```python
from build123d import *

# Parameters (mm, degrees)
SKETCH1_R           = 0.627
BOSS_EXTRUDE1_DEPTH = 0.762
FILLET1_R           = 2.54
FILLET2_RADIUS      = 0.5039995
FILLET2_LENGTH      = 0.762


with BuildPart() as part:
    # Sketch1 → Boss-Extrude1 (new body)
    with BuildSketch(Plane.XY):
        with BuildLine():
            Line((-0.508, -9.511443686), (-0.508, -17.4625))
            Line((-0.508, -17.4625), (0.499999, -17.4625))
            Line((0.499999, -17.4625), (0.499999, -9.51186764))
            ThreePointArc((0.499999, -9.51186764), (0.004006112, 9.524999158), (-0.508, -9.511443686))
        make_face()
        Circle(SKETCH1_R, mode=Mode.SUBTRACT)
    extrude(amount=BOSS_EXTRUDE1_DEPTH)

    # Fillet1
    fillet1_edges = [part.edges().sort_by_distance(p)[0] for p in [
        (0.499999, -9.51186764, 0.381),
        (-0.508, -9.511443686, 0.381),
    ]]
    fillet(fillet1_edges, radius=FILLET1_R)

    # Fillet2: full round fillet: the end face becomes a half cylinder, R = half its width
    fillet2_face = Plane((-0.0040005, -17.4625, 0.381), x_dir=(0, 0, 1), z_dir=(0, -1, 0))  # on the end face: x along it, z out of the body
    fillet2_slab = fillet2_face.offset(-FILLET2_RADIUS / 2) * Box(FILLET2_LENGTH, 2 * FILLET2_RADIUS, FILLET2_RADIUS, mode=Mode.PRIVATE)  # the body's end, R deep
    fillet2_round = Plane((-0.0040005, -16.9585005, 0.381), x_dir=(0, -1, 0), z_dir=(0, 0, 1)) * Cylinder(FILLET2_RADIUS, FILLET2_LENGTH, mode=Mode.PRIVATE)  # its axis R under the face
    add(fillet2_slab - fillet2_round, mode=Mode.SUBTRACT)


solid = part.part
```
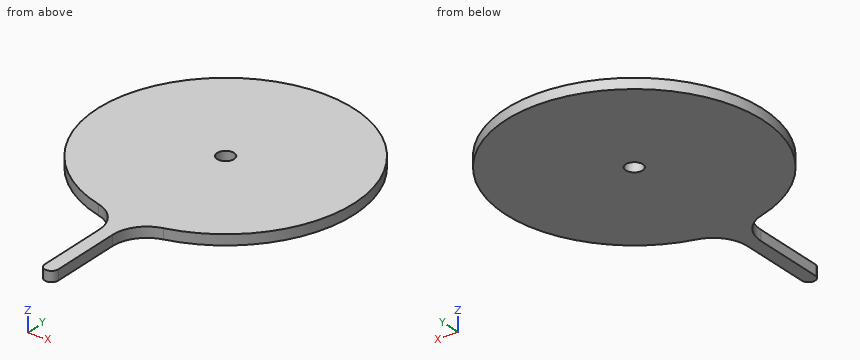
Geometry check sheet. Reference: the model listing, model coordinates, mm. Coordinates: 2 decimals unless noted, no trailing zeros. Order: outer loops, then holes, each group sorted by start corner. A loop starts at its lowest first (then second) coordinate and runs counter-clockwise, first axis right, second up.
Q1. Thickness scan on probe 1 along Y at (x, z) = (0, 0.3) (3 decimals); probe 2 along X at (y, z) = (-13.5, 0.2); probe 3 along X at (y, z) = (-0.5, 0.35). Record the ranges inside material, lowest first.
Reply:
probe 1: y = -17.462 to -0.627, 0.627 to 9.525
probe 2: x = -0.51 to 0.5
probe 3: x = -9.51 to -0.38, 0.38 to 9.51
Q2. Sectioned sample at A-A on y = 0. Record the cut outline in (x, z) (3 decimals), and give its area (3 significant figures).
Reply:
outline: (-9.525, 0) - (-0.627, 0) - (-0.627, 0.762) - (-9.525, 0.762) - close; (0.627, 0) - (9.525, 0) - (9.525, 0.762) - (0.627, 0.762) - close
area: 13.6 mm2
Q3. Sectioned sample at C-C on x = 0. Record the cut outline in (y, z) (3 decimals), and give its area (3 significant figures).
Reply:
outline: (-17.462, 0) - (-0.627, 0) - (-0.627, 0.762) - (-17.462, 0.762) - close; (0.627, 0) - (9.525, 0) - (9.525, 0.762) - (0.627, 0.762) - close
area: 19.6 mm2
Q4. Depth check by flat-ended pin: pin 1 Ø0.8 at (x, y) = (0, 0) entering from -Z. Enter the tip coordinate at first touch or a pass-through.
Reply:
pin 1: passes through
Q5. Sectioned sample at D-D on x = -3.25. Record the cut outline in (y, z), and give its area (3 significant figures).
Reply:
outline: (-8.95, 0) - (8.95, 0) - (8.95, 0.76) - (-8.95, 0.76) - close
area: 13.6 mm2
